The model under review builds one solid part; all positions refer to its coordinate system, in mm. A direction names the side the tool comes from. Coordinates: 2 decimals unless noted, no trailing zeros. Loops run counter-clockwise (first coordinate to the right, second up) from the corner with the lowest first, then second, coordinate; pieces in that order, holes last. Notation, with made-up numbers: (73.25, 54) - (100.25, 54) arc R17 ccw to (100.25, 87) - close; hole circle Ø5 at (69, -11.5). An arc over 180 degrees is marked (long way). Use a Markdown table: item, result. Add a question column.
1) Add section C-C, the plane x = 7.5. Give the boundary of the cut face in (y, z).
2) Clearance check with flat-ended pins moving along their axes: pin 1 (1 mm diameter, centred on x = 5, y = -1.5, fed in from +Z); pin 2 (1.5 mm diameter, centred on x = 2, z = -1.5, fed in from -Y); pin 3 (1.5 mm diameter, centred on y = 2.5, z = -4, fed in from +X); pin 4 (2 mm diameter, centred on x = 2, y = 1, fed in from +Z). State where each tip first meets the part, or that it passes through.
3) To check wall thickness, follow L1, parallel to Y at x = 6.25, z = -4.75; L2, parallel to Z at x = 6, y = -1.25; L3, parallel to Y at x = 3.5, z = -4.75. State the ranges of each line that lie inside material, in increasing order. Write a range as [from, to].
4) The part is to be moulded in two halves that separate along Z. For faces 4 (the flat face through (7.7, 1.5, -4.1)), 5 (the cylindrical face through (4.541, 0.394, -5.467)), 6 (the flat face through (3.9, 1.5, -7.7)), say which applies: pulls with the +Z half, pulls with the -Z half, needs draft (parallel to the pull), parting line crosses it, or undercut.
5) For faces 1 (the flat face through (4, -1, -7)), 2 (the flat face through (4, 0.8, -4)), 3 (the flat face through (5.164, 2.803, -4.17)), list the 3-axis set-ups (+Z, -Z, +X, -X, +Y, -Y) from which the entire face can be reached by the end or side of a thin tool; tool diameter is ignored.
6) Add section A-A, the plane y = 0.5. Give the boundary of the cut face in (x, z), and give its area (3 significant figures).
7) Add section B-B, the plane z = -2.75. Give the boundary of the cut face in (x, y).
8) Add section D-D, the plane y = 1.55. Give the boundary of the cut face in (x, z).
```python
from build123d import *

# Parameters (mm, degrees)
SKETCH1_W               = 8
SKETCH1_H               = 8
BOSS_EXTRUDE1_DEPTH     = 3
CUT_EXTRUDE1_DEPTH      = 12.704699911
CUT_EXTRUDE1_DEPTH_BACK = 12.704699911
CUT_EXTRUDE2_DEPTH      = 11
SKETCH4_R               = 1.8
CUT_EXTRUDE3_DEPTH      = 0.8
SKETCH5_W               = 8
SKETCH5_H               = 1
BOSS_EXTRUDE2_DEPTH     = 2
FILLET1_R               = 4
CUT_EXTRUDE4_DEPTH      = 0.4
CUT_EXTRUDE5_DEPTH      = 0.4


with BuildPart() as part:
    # Sketch1 → Boss-Extrude1 (new body)
    with BuildSketch(Plane(origin=(0, 0, 0), x_dir=(1, 0, 0), z_dir=(0, 1, 0))):
        with Locations((4, 4)):
            Rectangle(SKETCH1_W, SKETCH1_H)
    extrude(amount=BOSS_EXTRUDE1_DEPTH)

    # Sketch2 → Cut-Extrude1 (cut, two sides: drawn at the far end of the back side and taken through both)
    with BuildSketch(Plane.XY.offset(-CUT_EXTRUDE1_DEPTH_BACK)):
        Polygon((0, 0), (0.6, 3), (0, 3), align=None)
        Polygon((8, 0), (7.4, 3), (8, 3), align=None)
    extrude(amount=CUT_EXTRUDE1_DEPTH + CUT_EXTRUDE1_DEPTH_BACK, mode=Mode.SUBTRACT)

    # Sketch3 → Cut-Extrude2 (cut)
    with BuildSketch(Plane(origin=(0, 0, 0), x_dir=(0, 0, -1), z_dir=(1, 0, 0))):
        Polygon((0, 0), (0.6, 3), (0, 3), align=None)
        Polygon((8, 3), (7.4, 3), (8, 0), align=None)
    extrude(amount=CUT_EXTRUDE2_DEPTH, mode=Mode.SUBTRACT)

    # Sketch4 → Cut-Extrude3 (cut)
    with BuildSketch(Plane.XZ):
        with Locations(Location((4, -3.75, 0), (0, 0, 270))):
            Circle(SKETCH4_R)
    extrude(amount=-CUT_EXTRUDE3_DEPTH, mode=Mode.SUBTRACT)

    # Sketch5 → Boss-Extrude2 (add)
    with BuildSketch(Plane.XZ):
        with Locations((4, -7.5)):
            Rectangle(SKETCH5_W, SKETCH5_H)
    extrude(amount=BOSS_EXTRUDE2_DEPTH)

    # Fillet1
    # the kernel refuses this fillet: 4 mm, written as the material it takes off along each edge
    with BuildSketch(Plane(origin=(8, -2, -16.660254038), x_dir=(0, 1, 0), z_dir=(0, 0, 1)), Plane(origin=(0, -2, 1.660254038), x_dir=(0, 1, 0), z_dir=(0, 0, -1))) as fillet1_piece_1:
        with BuildLine():
            CenterArc((4, 3.464101615), FILLET1_R, 180, 60)
            Line((0, 3.464101615), (-0.08, 3.464101615))
            Line((-0.08, 3.464101615), (-0.08, 0))
            Line((-0.08, 0), (0, -0.08))
            ThreePointArc((0, -0.08), (1, -0.08), (1.96, -0.069282032))
            Line((1.96, -0.069282032), (2, 0))
        make_face()
    extrude(amount=18.320508076, mode=Mode.SUBTRACT)

    # Sketch6 → Cut-Extrude4 (cut)
    with BuildSketch(Plane(origin=(0, 3, 0), x_dir=(1, 0, 0), z_dir=(0, 1, 0))):
        Polygon((5.933857302, 2.141652068), (5.118152174, 2.141652068), (4.780812431, 3.064728992), (3.24555602, 3.064728992), (2.908216277, 2.141652068), (2.087703456, 2.141652068), (3.599722687, 6.141652068), (4.414626533, 6.141652068), align=None)
        Polygon((4.536421405, 3.731395658), (4.010780379, 5.167293094), (3.486741918, 3.731395658), align=None, mode=Mode.SUBTRACT)
    extrude(amount=-CUT_EXTRUDE4_DEPTH, mode=Mode.SUBTRACT)

    # Sketch7 → Cut-Extrude5 (cut)
    with BuildSketch(Plane(origin=(0, 3, 0), x_dir=(1, 0, 0), z_dir=(0, 1, 0))):
        Polygon((7.095591712, 1.44126633), (6.864822481, 1.44126633), (6.480207097, 1.85152274), (6.916104533, 1.85152274), align=None)
    extrude(amount=-CUT_EXTRUDE5_DEPTH, mode=Mode.SUBTRACT)


solid = part.part
```
From the geometry:
| question | item | result |
|---|---|---|
| 1 | outline | (-0.69, -8) - (0, -8) - (2.5, -7.5) - (2.5, -0.5) - (0, 0) - (0, -7) - (-0.69, -7) - close |
| 2 | pin 1 | stops at z = -7 |
| 2 | pin 2 | stops at y = 0 |
| 2 | pin 3 | stops at x = 7.65 |
| 2 | pin 4 | stops at z = 0 |
| 3 | L1 | y = [0, 3] |
| 3 | L2 | z = [-8, -7] |
| 3 | L3 | y = [0.8, 2.6] |
| 4 | face 4 | needs draft |
| 4 | face 5 | undercut |
| 4 | face 6 | pulls with the -Z half |
| 5 | face 1 | +Z, +X, -X, -Y |
| 5 | face 2 | -Y |
| 5 | face 3 | +Y |
| 6 | outline | (0.1, -7.9) - (7.9, -7.9) - (7.9, -0.1) - (0.1, -0.1) - close; hole circle Ø3.6 at (4, -3.75) |
| 6 | area | 50.7 mm^2 |
| 7 | outline | (0, 0) - (2.5, 0) - (2.5, 0.8) - (5.5, 0.8) - (5.5, 0) - (8, 0) - (7.4, 3) - (5.7, 3) - (5.7, 2.6) - (4.9, 2.6) - (4.9, 3) - (3.13, 3) - (3.13, 2.6) - (2.32, 2.6) - (2.32, 3) - (0.6, 3) - close |
| 8 | outline | (0.31, -7.69) - (7.69, -7.69) - (7.69, -0.31) - (0.31, -0.31) - close |
